Autodesk Inventor part; units mm, degrees
ref_plane "IDS_WORKPLANE{1}" through (0, 100, 0) normal (0, 1, 0) x (-1, 0, 0)
ref_plane "YZ Plane" through (0, 0, 0) normal (1, 0, 0) x (0, 1, 0)
ref_plane "XZ Plane" through (0, 0, 0) normal (0, 1, 0) x (-1, 0, 0)
sketch "Szkic1" plane through (0, 0, 0) normal (0, 0, 1) x (1, 0, 0)
  line L0 (0, 100) -> (28, 100)
  line L1 (-1.9497, 0) -> (21.5466, 0)
  line L2 (0, 100) -> (0, 75)
  line L3 (0, 75) -> (28, 75)
  line L4 (28, 75) -> (28, 100)
  line L5 (-6.6489, 0) -> (26.2458, 0)
  line L6 (0, 48) -> (0, -8)
  dimension "d0" = 200
  dimension "d1" = 150
  dimension "d2" = 28
revolve "Bryła" add sketch "Szkic1" angle 360 about axis through (-1.9497, 0, 0) along (1, 0, 0)
ref_plane "IDS_WORKPLANE{1}" through (0, 100, 0) normal (0, 1, 0) x (-1, 0, 0)
sketch "Szkic2" plane through (0, 100, 0) normal (0, 1, 0) x (-1, 0, 0)
  line L0 (0, 100) -> (0, -100)
  line L1 (-10.8, 0) -> (1.8, 0)
  point P0 (-14, 0)
  dimension "d7" = 14
hole "Otwór1" at (14, 100, 0) direction (0, -1, 0) diameter 16 end up to surface
chamfer "Faza1" distance 2.8 angle 45 1 edges at (28, -100, 0) measured on face at (9.3333, 87.1784, -48.989)
equation "\"d8\" = NND"
equation "\"d4\" = PHH"
equation "\"d5\" = FAWI"
equation "\"d22\" = PHH"
equation "\"d0\" = SD2"
equation "\"d1\" = WND"
equation "\"d2\" = SD"
equation "\"WND\" = 150"
equation "\"SD2\" = 200"
equation "\"SD\" = 28"
equation "\"NND\" = 16"
equation "\"FAWI\" = 45deg"
equation "\"PHH\" = 2.8"
properties part number "DIN 705 - B150" material "Stal, miękka"
Build history of the part. All positions in model axes, mm. A direction names the side the tool comes from. Round coordinates to 2 decimals unless told otherwise and drop trailing zeros. Write each loop counter-clockwise with the first axis right and the second up, starting at its lowest first coordinate (ties: lowest second). Pieces come first, ordered by that corner, then holes. Notation, with made-up numbers: M 24.25,46 L 81.25,46 A22 cw 81.25,80 Z; hole C -1.75,62 d8. An arc over 180 degrees is marked long. Use CSV: the item, a comma, the result in double quotes.
1. Wall check: probe 1 along Z at (x, y) = (21.25, 0); probe 2 along Z at (x, y) = (11.75, -42); probe 3 along Y at (x, z) = (18, -63.5). Give the ranges that are in metal, low to high. Write a range as from..to.
Reply:
probe 1,"z = -100..-75, 75..100"
probe 2,"z = -90.75..-62.14, 62.14..90.75"
probe 3,"y = -77.25..-39.91, 39.91..77.25"
2. Tool access for faces 1 (the face through (27.825, -77.274, 59.251)), 2 (the face through (8.6, 87.1, -5.9)): list every direction of +Z, -Z, +X, -X, +Y, -Y with a clear straight run to the whole face (end or side of a thin tool).
Reply:
face 1,"+X"
face 2,"+Y"
3. Flat gauge pins, fed straight in: pin 1 (2 mm diameter, centred on y = 39.5, z = -61.5, fed in from +X); pin 2 (12 mm diameter, centred on x = 14, y = -10, fed in from +Z); pin 3 (2 mm diameter, centred on x = 24, y = -68.5, fed in from -Z); pin 4 (6 mm diameter, centred on x = 10.5, z = 22.5, fed in from +Y). Where does each tip first touch, or does it go through?
Reply:
pin 1,"passes through"
pin 2,"stops at z = 99.92"
pin 3,"stops at z = -73.78"
pin 4,"stops at y = 98.08"
4. Saw through at C-C (x = 8.75). Give the cut face in (y, z).
Reply:
outline,"M 74.76,-6.04 A75 cw long 74.76,6.04 L 99.82,6.04 A100 ccw long 99.82,-6.04 Z"
5. Two-plate mould, pull along Y, no slides. Class faces 3 (the face through (0, 14, 75)), 4 (the face through (14.196, -9.764, 74.362)), 5 (the face through (12.78, 95.38, 30.04)): +Y half, -Y half, draft (parallel to the pull), parting line (faces both ways), or undercut.
Reply:
face 3,"draft"
face 4,"undercut"
face 5,"parting line"
6. Saw through at A-A (y = 0). Give the cut face in (x, z), plus the area to 3 significant figures.
Reply:
outline,"M 0,-100 L 25.2,-100 L 28,-97.2 L 28,-75 L 0,-75 Z; M 0,75 L 28,75 L 28,97.2 L 25.2,100 L 0,100 Z"
area,"1,390 mm²"
7. Saw through at B-B (z = 0). Give the cut face in (x, y).
Reply:
outline,"M 0,-100 L 25.2,-100 L 28,-97.2 L 28,-75 L 0,-75 Z; M 0,75 L 6,75 L 6,100 L 0,100 Z; M 22,75 L 28,75 L 28,97.2 L 25.2,100 L 22,100 Z"
